Autodesk Inventor part; units mm, degrees
ref_plane "YZ Plane" through (0, 0, 0) normal (1, 0, 0) x (0, 1, 0)
ref_plane "XZ Plane" through (0, 0, 0) normal (0, 1, 0) x (-1, 0, 0)
ref_plane "XY Plane" through (0, 0, 0) normal (0, 0, 1) x (1, 0, 0)
sketch "Sketch2" plane through (0, 0, 0) normal (1, 0, 0) x (0, 1, 0)
  line L0 (18.4798, 0) -> (-23.1628, 0)
  line L1 (0, 0) -> (-11, 0) construction
  line L2 (-11, 0) -> (-11, -50) construction
  line L3 (-11, -50) -> (0, -50) construction
  line L4 (0, -50) -> (0, 0) construction
  line L5 (0.7575, -40) -> (-11, -40) construction
  line L6 (35.6298, -95) -> (-28.9625, -95) construction
  line L7 (0, -50) -> (-11, -50)
  line L8 (-11, -50) -> (-11, -58)
  line L9 (-11, -58) -> (0, -58)
  line L10 (0, -58) -> (0, -50)
  line L11 (3, -47.5) -> (0, -47.5)
  line L12 (0, -47.5) -> (0, -72.5)
  line L13 (0, -72.5) -> (3, -72.5)
  line L14 (3, -72.5) -> (3, -47.5)
  dimension "d9" = 100
  dimension "d10" = 11
  dimension "d11" = 10
  dimension "d12" = 190
  dimension "d13" = 8
  dimension "d14" = 2.5
  dimension "d15" = 3
  dimension "d16" = 25
revolve "Revolution3" add sketch "Sketch2" angle 360 about axis through (0, 18.4798, 0) along (0, -1, 0)
sketch "Sketch3" plane through (0, -11, 0) normal (0, -1, 0) x (1, 0, 0)
  circle A0 centre (0, 0) radius 50
  line L0 (0, 0) -> (103.1518, 0)
  circle A1 centre (52.25, 0) radius 4.75
  circle A2 centre (52.25, 0) radius 1.6
  arc A3 (46.338, -10.4421) -> (45.9796, 11.9216) centre (0, 0) ccw construction
  dimension "d19" = 9.5
  dimension "d20" = 3.2
  dimension "d25" = 2.5
extrude "Extrusion1" cut sketch "Sketch3" against normal through all contours A2 L0 | L0 A2
extrude "Extrusion2" cut sketch "Sketch3" against normal blind 1 contours L0 A1 A0 | L0 A2 A1 A0 | A0 A1 L0 | A0 A1 L0 A2
pattern_circular "Circular Pattern1" count 6 over 360 about axis through (0, 1.5, 0) along (0, -1, 0) of "Extrusion1", "Extrusion2"
sketch "Sketch4" plane through (0, 3, 0) normal (0, 1, 0) x (1, 0, 0)
  point P0 (0, 0)
sketch "Sketch5" plane through (0, 3, 0) normal (0, 1, 0) x (1, 0, 0)
  circle A0 centre (0, 0) radius 47.5
  line L0 (0, 0) -> (0, 79.7699)
  circle A1 centre (-7.5, 55) radius 1.6
  line L1 (0, 0) -> (104.7189, 0)
  circle A2 centre (-7.5, 65) radius 1.6
  circle A3 centre (7.5, 55) radius 1.6
  circle A4 centre (7.5, 65) radius 1.6
  dimension "d29" = 3.2
  dimension "t" = 7.5
  dimension "d31" = 55
  dimension "d34" = 10
  dimension "d37" = 15
extrude "Extrusion3" cut sketch "Sketch5" against normal through all contours A1 | A2 | A3 | A4
pattern_circular "Circular Pattern2" count 6 over 360 about axis through (0, 1.5, 0) along (0, -1, 0) of "Extrusion3"
sketch "Sketch6" plane through (0, -11, 0) normal (0, -1, 0) x (1, 0, 0)
  circle A0 centre (43.8814, -33.9952) radius 1.6
  circle A1 centre (51.3814, -21.0048) radius 1.6
  circle A2 centre (43.8814, -33.9952) radius 3.25
  circle A3 centre (51.3814, -21.0048) radius 3.25
  point P0 (0, 0)
  dimension "d45" = 6.5
  dimension "d46" = 6.5
extrude "Extrusion4" cut sketch "Sketch6" against normal up to surface (11 mm away)
pattern_circular "Circular Pattern3" count 6 over 360 about axis through (0, -5.5, 0) along (0, -1, 0) of "Extrusion4"
equation "\"d37\" = 2 * t"
properties part number "rotor-case"
Work out the finished part from the listing and answer in its coordinate system (mm). A direction names the side the tool comes from. Give positions to 0.01 mm unless a question says otherwise; leave off trailing zeros. Loops run counter-clockwise (first coordinate to the right, second up) from the corner with the lowest first, then second, coordinate; pieces in that order, holes last. Notation, with made-up numbers: (81.5, -17.5) -> (87.5, -17.5) arc R27 ccw to (87.5, 4.5) -> close; hole circle Ø6 at (32, 5.25). An arc over 180 degrees is marked (long way). Use a Markdown table: item, result. Add a question column.
1) The part is cut by section B-B, the plane y = -4.25. Count the separate pieces of the cut face and the enclosed holes in it, plus the area to 3 significant figures.
2) Which of the six approach directions +Z, -Z, +X, -X, +Y, -Y give full straight-line access (tool end or side, diameter ignored) to faces 1 (the cylindrical face through (0, -5, 58)), 2 (the cylindrical face through (-28.38, -10.51, 49.43)), 3 (the cylindrical face through (-50.943, 1.521, -38.925))?
3) Each of these flat-tipped pins is pushed along its axis until it touches: P1, Ø8.5, axis at x = 51.38, z = 21, coming from the -Y side; P2, Ø3, axis at x = -30, y = -5.5, coming from the +Z side; P3, Ø1.5, axis at x = 32.5, y = -3.5, coming from the +Z side; P4, Ø1, axis at y = -7.5, z = 7, coming from the +X side. Where does it stop, or does it pass through?
4) For a pull along Z with two mould halves and no side action, classify faces 4 (the cylindrical face through (50.27, -5.42, -28.93)), 5 (the flat face through (-43, -11, 26)), 6 (the cylindrical face through (-41.25, -5.58, -32.09)) as +Z half, -Z half, draft (parallel to the pull), parting line (faces both ways), or undercut.
5) The part is cut by section C-C, the plane x = 36.5. Determine the outline of the cut face in (y, z).
6) The part is cut by section A-A, the plane x = 0. Determine the outline of the cut face in (y, z), plus the area to 3 significant figures.
7) Consider line 1 along Z through (x, y) = (-44, 0.5); line 2 along Z through (x, y) = (-43.5, -7.75); line 3 along Z through (x, y) = (-60, 1.5). Determine where each line is inside the solid, lowest interval first.
Reported:
| question | item | result |
|---|---|---|
| 1 | separate pieces | 1 |
| 1 | enclosed holes | 7 |
| 1 | area | 2,290 mm^2 |
| 2 | face 1 | +Z, -Y |
| 2 | face 2 | -Y |
| 2 | face 3 | +Y, -Y |
| 3 | P1 | stops at y = -11 |
| 3 | P2 | stops at z = 50.51 |
| 3 | P3 | stops at z = 48.54 |
| 3 | P4 | stops at x = 57.63 |
| 4 | face 4 | -Z half |
| 4 | face 5 | draft |
| 4 | face 6 | undercut |
| 5 | outline | (-11, -45.07) -> (0, -45.07) -> (0, -62.64) -> (3, -62.64) -> (3, -30.4) -> (0, -30.4) -> (0, -34.17) -> (-11, -34.17) -> close; (-11, 34.17) -> (0, 34.17) -> (0, 30.4) -> (3, 30.4) -> (3, 62.64) -> (0, 62.64) -> (0, 45.07) -> (-11, 45.07) -> close |
| 6 | outline | (-11, -58) -> (0, -58) -> (0, -72.5) -> (3, -72.5) -> (3, -47.5) -> (0, -47.5) -> (0, -50) -> (-11, -50) -> close; (-11, 50) -> (0, 50) -> (0, 47.5) -> (3, 47.5) -> (3, 72.5) -> (0, 72.5) -> (0, 58) -> (-11, 58) -> close |
| 6 | area | 326 mm^2 |
| 7 | line 1 | z = -57.62 to -35.59, -32.4 to -17.9, 17.9 to 32.4, 35.59 to 57.62 |
| 7 | line 2 | z = -38.36 to -37.22, -30.77 to -24.65, 24.65 to 30.77, 37.22 to 38.36 |
| 7 | line 3 | z = -40.7 to -27.6, -24.41 to 24.41, 27.6 to 40.7 |
